```python
from build123d import *

# Parameters (mm, degrees)
F0_W     = 1828.8
F0_H     = 330.2
F1_DEPTH = 76.2
F2_W     = 25.4
F2_H     = 25.4
F3_DEPTH = 838.2
F4_W     = 25.4
F4_H     = 25.4
F5_DEPTH = 1746.25
F6_W     = 25.4
F6_H     = 25.4
F7_DEPTH = 215.9


with BuildPart() as f1:
    # F0 (on Top) → F1 (new body)
    with BuildSketch(Plane.XY):
        Rectangle(F0_W, F0_H)
        Polygon((-914.4, -165.1), (-914.4, 165.1), (-1016, 165.1), align=None)
        Polygon((1016, 165.1), (914.4, 165.1), (914.4, -165.1), align=None)
    extrude(amount=F1_DEPTH)

    # F2 (on face) → F3 (join)
    with BuildSketch(Plane(origin=(0, 0, 0), x_dir=(1, 0, 0), z_dir=(0, 0, -1))):
        with Locations((885.825, 114.3)):
            Rectangle(F2_W, F2_H)
        with Locations((-885.825, 114.3)):
            Rectangle(F2_W, F2_H)
        with Locations((-885.825, -127)):
            Rectangle(F2_W, F2_H)
        with Locations((885.825, -127)):
            Rectangle(F2_W, F2_H)
    extrude(amount=F3_DEPTH)

    # F4 (on face) → F5 (join, through all)
    with BuildSketch(Plane.YZ.offset(-873.125)):
        with Locations((127, -825.5)):
            Rectangle(F4_W, F4_H)
    extrude(amount=F5_DEPTH)

    # F6 (on face) → F7 (join, through all)
    with BuildSketch(Plane.XZ.offset(-114.3)):
        with Locations((885.825, -825.5)):
            Rectangle(F6_W, F6_H)
        with Locations((-885.825, -825.5)):
            Rectangle(F6_W, F6_H)
    extrude(amount=F7_DEPTH)


solid = f1.part
```
Here's how the part is built. I have some questions about the finished solid (model axes, mm). A direction names the side the tool comes from. Give positions to 0.01 mm unless a question says otherwise; leave off trailing zeros. Order: outer loops, then holes, each group sorted by start corner. A loop starts at its lowest first (then second) coordinate and runs counter-clockwise, first axis right, second up. Notation, with made-up numbers: (-30.5, 63.25) -> (6.5, 63.25) arc R7 ccw to (6.5, 71.25) -> close; hole circle Ø8 at (-17, 13.25). An arc over 180 degrees is marked (long way). Use CSV: the item, a comma, the result in double quotes. Start each with the question number.
Item 1: I'm going to push flat-ended pins straight in: P1, Ø7.5, axis at x = 112.5, z = -824, coming from the -Y side; P2, Ø7.5, axis at x = -888, z = -410, coming from the -Y side; P3, Ø8, axis at y = 118, z = -237.5, coming from the -X side (3 decimals). Where does each tip first touch, or does it pass through?
Item 2: Suppose I cut it at A-A (y = -19.5). List the corners of the cut face in (x, z) for me (3 decimals).
Item 3: If I drill on probe 1 along Z at (x, y) = (-304, 117); probe 2 along X at (y, z) = (120.5, -411.5) (3 decimals); probe 3 along Z at (x, y) = (-545.5, -148), over which ranges is the centre line in solid material (lowest first)? Write a range as [from, to].
Item 4: Thinking about a two-plate mould opening in X: for faces 1 (the flat face through (-873.125, -104, -514)), 2 (the flat face through (-965.91, 2.31, 37.57)), 3 (the flat face through (964.49, -2.31, 37.57)), 4 (the flat face through (-4, 139.7, -825)), which applies, pulls with the +X half, pulls with the -X half, needs draft (parallel to the pull), parting line crosses it, or undercut?
Item 5: On a 3-axis mill with a long thin cutter (end or side, diameter ignored), from which of +Z, -Z, +X, -X, +Y, -Y can I reach the whole of each face in a straight line? I mean faces 5 (the flat face through (873.125, -104, -514)), 6 (the flat face through (898.525, -102, -483)), 7 (the flat face through (14, 165.1, 38)), 8 (the flat face through (-898.525, -102, -448)). Say none if no direction works.
Item 6: Suppose I cut it at B-B (x = -516.5). List the corners of the cut face in (y, z) for me, and give its area (3 significant figures).
Item 7: Suppose I cut it at C-C (z = -62.5). List the corners of the cut face in (x, y) for me (3 decimals).
Answer block:
1,P1,"stops at y = 114.3"
1,P2,"stops at y = -127"
1,P3,"stops at x = -898.525"
2,outline,"(-959.2, 0) -> (959.2, 0) -> (959.2, 76.2) -> (-959.2, 76.2) -> close; (-898.525, -838.2) -> (-873.125, -838.2) -> (-873.125, -812.8) -> (-898.525, -812.8) -> close; (873.125, -838.2) -> (898.525, -838.2) -> (898.525, -812.8) -> (873.125, -812.8) -> close"
3,probe 1,"z = [-838.2, -812.8], [0, 76.2]"
3,probe 2,"x = [-898.525, -873.125], [873.125, 898.525]"
3,probe 3,"z = [0, 76.2]"
4,face 1,"undercut"
4,face 2,"pulls with the -X half"
4,face 3,"pulls with the +X half"
4,face 4,"needs draft"
5,face 5,"-Z, -Y"
5,face 6,"-Z, +X, +Y, -Y"
5,face 7,"+Z, -Z, +X, -X, +Y"
5,face 8,"-Z, -X, +Y, -Y"
6,outline,"(-165.1, 0) -> (165.1, 0) -> (165.1, 76.2) -> (-165.1, 76.2) -> close; (114.3, -838.2) -> (139.7, -838.2) -> (139.7, -812.8) -> (114.3, -812.8) -> close"
6,area,"25,800 mm^2"
7,outline,"(-898.525, -127) -> (-873.125, -127) -> (-873.125, -101.6) -> (-898.525, -101.6) -> close; (-898.525, 114.3) -> (-873.125, 114.3) -> (-873.125, 139.7) -> (-898.525, 139.7) -> close; (873.125, -127) -> (898.525, -127) -> (898.525, -101.6) -> (873.125, -101.6) -> close; (873.125, 114.3) -> (898.525, 114.3) -> (898.525, 139.7) -> (873.125, 139.7) -> close"
